The listing builds one solid part. Answer for the finished solid, in the listing's coordinates (mm). Face numbers are marked on the shaded views. A direction names the side the tool comes from. Round coordinates to 2 decimals unless told otherwise and drop trailing zeros. Order: outer loops, then holes, each group sorted by start corner. A loop starts at its lowest first (then second) coordinate and runs counter-clockwise, first axis right, second up. Notation, with made-up numbers: M 64.25,-4 L 104.25,-4 A25 cw 104.25,12 Z; hole C 70,-22.75 d9. An arc over 180 degrees is marked long. Write item = value, one per line. Start each with the question number.
(1) Straight lines are drawn through the part: probe 1 along Y at (x, z) = (0, 2.25) (3 decimals); probe 2 along X at (y, z) = (17.5, 5); probe 3 along Y at (x, z) = (-17.78, 3.25). For each, find the intervals that lie inside material, in ascending order. Write a range as from..to.
(2) For a pull along Y with two mould halves and no side action, classify the marked faces 1, 2 and 3 as released by +Y, released by -Y, zero draft, split by the parting line, or undercut.
(3) A cutting plane is placed at B-B, the plane z = 10.5. Determine the outline of the cut face in (x, y) (3 decimals), and give its area (3 significant figures).
(4) Which of the six approach directions +Z, -Z, +X, -X, +Y, -Y give full straight-line access (tool end or side, diameter ignored) to the marked faces 4 and 5?
(5) A cutting plane is placed at D-D, the plane x = 14. Determine the outline of the cut face in (y, z), and give its area (3 significant figures).
(6) Each of these flat-tipped pins is pushed along its axis until it touches: pin 1 (2.5 mm diameter, centred on x = 17.78, y = 0, fed in from -Z); pin 2 (4 mm diameter, centred on y = 17, z = 7, fed in from +X); pin 3 (1.5 mm diameter, centred on y = 8.5, z = 4, fed in from -X). Where does it stop, or does it pass through?
(7) A cutting plane is placed at A-A, the plane z = 3. Determine the outline of the cut face in (x, y) (3 decimals), and give its area (3 significant figures).
(8) A cutting plane is placed at C-C, the plane y = 23. Determine the outline of the cut face in (x, z), and give its area (3 significant figures).
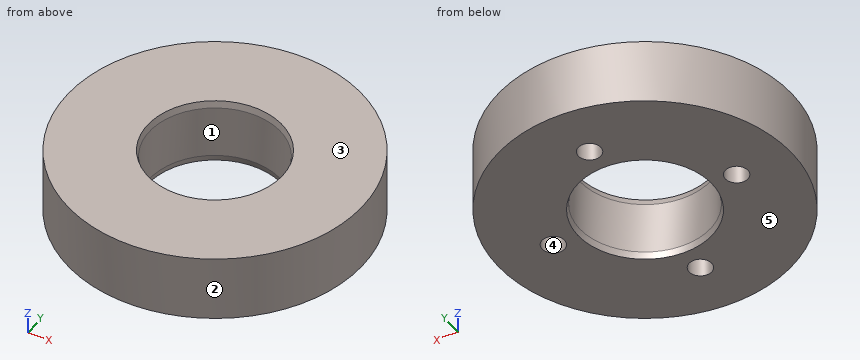
from build123d import *

# Parameters (mm, degrees)
F0_R     = 28.575
F0_R_2   = 12.7
F1_DEPTH = 12.7
F2_SIZE2 = 0.3402954744
F2_SIZE  = 1.27
F4_D     = 4.3942
F4_DEPTH = 6.35
F4_TIP   = 1.3201508661


with BuildPart() as f1:
    # F0 (on Top) → F1 (new body)
    with BuildSketch(Plane.XY):
        Circle(F0_R)
        Circle(F0_R_2, mode=Mode.SUBTRACT)
    extrude(amount=F1_DEPTH)

    # F2
    f2_edges = [f1.edges().sort_by_distance(p)[0] for p in [
        (-12.7, 0, 12.7),
        (-12.7, 0, 0),
    ]]
    f2_side = f1.faces().sort_by_distance((-12.7, 0, 6.35))[0]
    chamfer(f2_edges, length=F2_SIZE, length2=F2_SIZE2, reference=f2_side)

    # F4
    with Locations(Plane(origin=(0, 0, 0), x_dir=(1, 0, 0), z_dir=(0, 0, -1))):
        with Locations((0, -17.78), (-17.78, 0), (0, 17.78), (17.78, 0)):
            Hole(F4_D / 2, depth=F4_DEPTH)
            with Locations((0, 0, -(F4_DEPTH + F4_TIP / 2))):  # 118° drill point
                Cone(0, F4_D / 2, F4_TIP, mode=Mode.SUBTRACT)


solid = f1.part
Reported:
q1.probe_1 = -28.575..-19.977, -15.583..-12.7, 12.7..15.583, 19.977..28.575
q1.probe_2 = -22.59..-2.18, 2.18..22.59
q1.probe_3 = -22.37..-2.2, 2.2..22.37
q2.face_1 = undercut
q2.face_2 = split by the parting line
q2.face_3 = zero draft
q3.outline = C 0,0 d57.15; hole C 0,0 d25.4
q3.area = 2,060 mm²
q4.face_4 = -Z
q4.face_5 = -Z, +X, -X, +Y, -Y
q5.outline = M -24.91,0 L 24.91,0 L 24.91,12.7 L -24.91,12.7 Z
q5.area = 633 mm²
q6.pin_1 = 6.92
q6.pin_2 = 24.32
q6.pin_3 = -27.5
q7.outline = C 0,0 d57.15; hole C -17.78,0 d4.394; hole C 0,0 d25.4; hole C 0,-17.78 d4.394; hole C 0,17.78 d4.394; hole C 17.78,0 d4.394
q7.area = 2,000 mm²
q8.outline = M -16.96,0 L 16.96,0 L 16.96,12.7 L -16.96,12.7 Z
q8.area = 431 mm²
